For this review, use the dimensioned drawing (mm, ordinates from the lowest corner) and the shaded views. A direction names the side the tool comes from. Round coordinates to 2 decimals unless told otherwise and drop trailing zeros. Order: outer loops, then holes, each group sorted by start corner. A loop starts at its lowest first (then second) coordinate and runs counter-clockwise, first axis right, second up. Notation, with made-up numbers: (27.25, 23.25) -> (40.25, 23.25) arc R20 ccw to (40.25, 32.25) -> close; hole circle Ø5 at (20.25, 82.25). An arc over 180 degrees is marked (long way). Answer in a Markdown table with one row per item.
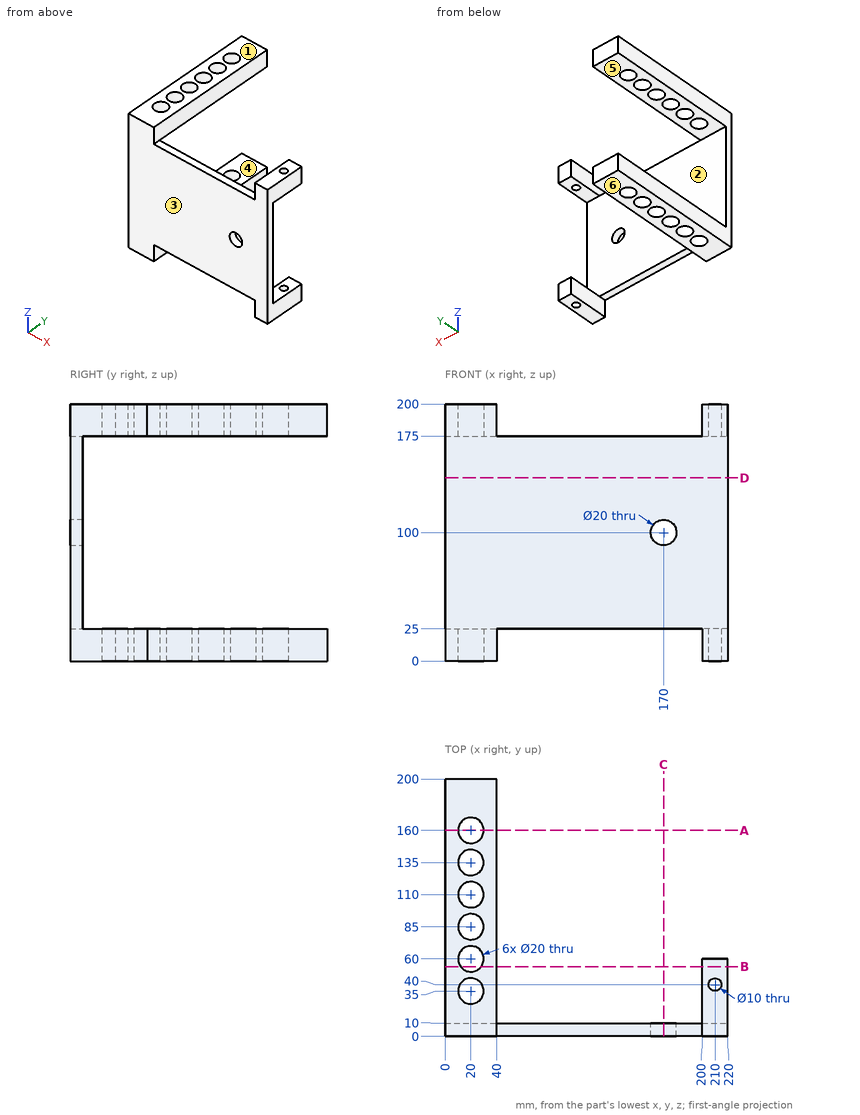
Q1. Take a section at D-D, the plane z = 142.5. Write out the cut boundary in (x, y), then the cut area to 3 significant figures.
Answer key:
| item | result |
|---|---|
| outline | (0, 0) -> (220, 0) -> (220, 10) -> (0, 10) -> close |
| area | 2,200 mm^2 |
Q2. To check wall thickness, follow probe 1 along Y at (x, z) = (210, 8.25); probe 2 along X at (y, z) = (153.5, 182.5); probe 3 along X at (y, z) = (4.5, 100). State the ranges of each line that lie inside material, in increasing order.
Answer key:
| item | result |
|---|---|
| probe 1 | y = 0 to 35, 45 to 60 |
| probe 2 | x = 0 to 12.4, 27.6 to 40 |
| probe 3 | x = 0 to 160, 180 to 220 |
Q3. Take a section at A-A, the plane y = 160. Write out the cut boundary in (x, z), then the cut area to 3 significant figures.
Answer key:
| item | result |
|---|---|
| outline | (0, 0) -> (10, 0) -> (10, 25) -> (0, 25) -> close; (0, 175) -> (10, 175) -> (10, 200) -> (0, 200) -> close; (30, 0) -> (40, 0) -> (40, 25) -> (30, 25) -> close; (30, 175) -> (40, 175) -> (40, 200) -> (30, 200) -> close |
| area | 1,000 mm^2 |
Q4. Take a section at B-B, the plane y = 54. Write out the cut boundary in (x, z), then the cut area to 3 significant figures.
Answer key:
| item | result |
|---|---|
| outline | (0, 0) -> (12, 0) -> (12, 25) -> (0, 25) -> close; (0, 175) -> (12, 175) -> (12, 200) -> (0, 200) -> close; (28, 0) -> (40, 0) -> (40, 25) -> (28, 25) -> close; (28, 175) -> (40, 175) -> (40, 200) -> (28, 200) -> close; (200, 0) -> (220, 0) -> (220, 25) -> (200, 25) -> close; (200, 175) -> (220, 175) -> (220, 200) -> (200, 200) -> close |
| area | 2,200 mm^2 |
Q5. Clearance check with flat-ended pins moving along their axes: pin 1 Ø23 at (x, z) = (170, 100) entering from +Y; pin 2 Ø22 at (x, z) = (213.5, 182.5) entering from +Y. State where each tip first meets the part, or that it passes through.
Answer key:
| item | result |
|---|---|
| pin 1 | stops at y = 10 |
| pin 2 | stops at y = 60 |
Q6. Tool access review of the marked faces 5 and 6: name each direction out of +Z, -Z, +X, -X, +Y, -Y from which nothing blocks a thin tool from reaching the whole face with its end or side.
Answer key:
| item | result |
|---|---|
| face 5 | +X, -X, +Y |
| face 6 | -Z, +X, -X, +Y, -Y |
Q7. Take a section at C-C, the plane x = 170. Write out the cut boundary in (y, z), then the cut area to 3 significant figures.
Answer key:
| item | result |
|---|---|
| outline | (0, 25) -> (10, 25) -> (10, 90) -> (0, 90) -> close; (0, 110) -> (10, 110) -> (10, 175) -> (0, 175) -> close |
| area | 1,300 mm^2 |
Q8. The part is to be moulded in two halves that separate along Z. For the marked faces 1, 2, 3 and 4, say which applies: +Z half, -Z half, draft (parallel to the pull), parting line (faces both ways), or undercut.
Answer key:
| item | result |
|---|---|
| face 1 | +Z half |
| face 2 | undercut |
| face 3 | draft |
| face 4 | undercut |
